from build123d import *

# Parameters (mm, degrees)
BOSS_EXTRUDE1_DEPTH = 33
SHELL1_T            = -10


with BuildPart() as part:
    # Sketch1 → Boss-Extrude1 (new body)
    with BuildSketch(Plane(origin=(0, 0, 0), x_dir=(1, 0, 0), z_dir=(0, 1, 0))):
        with BuildLine():
            ThreePointArc((81.419785193, -10.723465188), (1.062753422, 82.116043997), (-81.670036167, -8.612741664))
            ThreePointArc((-81.670036167, -8.612741664), (-53.746253944, -31.208811817), (-31.150183791, -3.285029594))
            ThreePointArc((-31.150183791, -3.285029594), (0.405350187, 31.320297905), (31.054734295, -4.090091387))
            ThreePointArc((31.054734295, -4.090091387), (52.920572843, -32.589303736), (81.419785193, -10.723465188))
        make_face()
    extrude(amount=BOSS_EXTRUDE1_DEPTH)

    # Shell1
    shell1_openings = [part.faces().sort_by_distance(p)[0] for p in [
        (-53.956492273, 0, 29.21523386),
    ]]
    offset(amount=SHELL1_T, openings=shell1_openings, kind=Kind.INTERSECTION)


solid = part.part
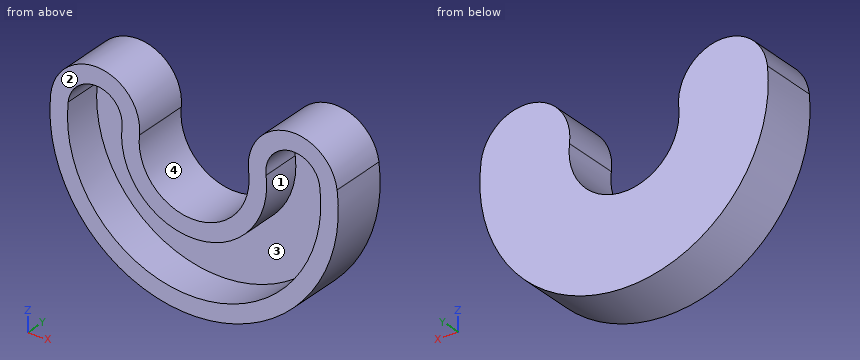
Verification items for the finished model (mm, model axes). Face numbers are marked on the shaded views. A direction names the side the tool comes from. Coordinates: 2 decimals unless noted, no trailing zeros. Write each loop counter-clockwise with the first axis right and the second up, starting at its lowest first coordinate (ties: lowest second). Pieces come first, ordered by that corner, then holes. Notation, with made-up numbers: (24, 42.25) - (44, 42.25) arc R23 ccw to (44, 71.25) - close; hole circle Ø1 at (35, 53). An arc over 180 degrees is marked (long way). Answer as a JSON object with one key per item and string values.
(1) Tool access check on the marked faces 3 and 4. Record the directions out of +Z, -Z, +X, -X, +Y, -Y that give a thin tool (end or side, any length) a straight path to the whole face; none if there is none.
Report:
{"face 3": "-Y", "face 4": "+Y, -Y"}
(2) Thickness scan on line 1 along Z through (x, y) = (0, 14.5); line 2 along X through (y, z) = (3, -13); line 3 along X through (y, z) = (20, 0). Record the ranges inside material, lowest first.
Report:
{"line 1": "-82.12 to -72.12, -41.32 to -31.32", "line 2": "-81.09 to -70.94, -39.22 to -28.5, 28.5 to 39.22, 70.94 to 81.09", "line 3": "-82.12 to -72.12, -41.32 to -31.32, 31.32 to 41.32, 72.12 to 82.12"}
(3) Cross-section at C-C on y = 3. Record the cut outline in (x, z), plus the area to 3 significant figures.
Report:
{"outline": "(-81.67, 8.61) arc R82.12 ccw (long way) to (81.42, 10.72) arc R25.4 ccw to (31.05, 4.09) arc R31.32 cw (long way) to (-31.15, 3.29) arc R25.4 ccw to start; hole (-71.73, 7.56) arc R72.12 ccw (long way) to (71.51, 9.42) arc R15.4 ccw to (40.97, 5.4) arc R41.32 cw (long way) to (-41.1, 4.33) arc R15.4 ccw to start", "area": "5,110 mm^2"}
(4) Gauge pin test, flat ends, axial feed: pin 1 Ø1 at (x, z) = (-36.5, -29.5) entering from -Y; pin 2 Ø5 at (y, z) = (7.5, -5.5) entering from -X; pin 3 Ø4 at (y, z) = (15.5, -57.5) entering from +X. Record the tip position at first contact, or that the pin passes through.
Report:
{"pin 1": "y = 23", "pin 2": "x = -82.07", "pin 3": "x = 60.53"}
(5) Cross-section at A-A on z = 0. Record the cut outline in (x, y), plus the area to 3 significant figures.
Report:
{"outline": "(-82.12, 0) - (-72.12, 0) - (-72.12, 23) - (-41.32, 23) - (-41.32, 0) - (-31.32, 0) - (-31.32, 33) - (-82.12, 33) - close; (31.32, 0) - (41.32, 0) - (41.32, 23) - (72.12, 23) - (72.12, 0) - (82.12, 0) - (82.12, 33) - (31.32, 33) - close", "area": "1,940 mm^2"}
(6) Cross-section at B-B on x = 0. Record the cut outline in (y, z), plus the area to 3 significant figures.
Report:
{"outline": "(0, -82.12) - (33, -82.12) - (33, -31.32) - (0, -31.32) - (0, -41.32) - (23, -41.32) - (23, -72.12) - (0, -72.12) - close", "area": "968 mm^2"}
(7) Cross-section at D-D on z = -63.5. Record the cut outline in (x, y), plus the area to 3 significant figures.
Report:
{"outline": "(-52.08, 0) - (-34.2, 0) - (-34.2, 23) - (34.2, 23) - (34.2, 0) - (52.08, 0) - (52.08, 33) - (-52.08, 33) - close", "area": "1,860 mm^2"}
(8) Mould release check, pull along Z, two halves, no side actions. Record for the marked faces 1 and 2: pulls with the +Z half, pulls with the -Z half, needs draft (parallel to the pull), parting line crosses it, or undercut.
Report:
{"face 1": "undercut", "face 2": "needs draft"}
